Autodesk Fusion 360 part; units mm, degrees
sketch "Sketch1" plane through (0, 0, 0) normal (0, 0, 1) x (1, 0, 0)
  line L0 (0, 0) -> (129, 0)
  line L1 (129, 0) -> (129, 96.5)
  line L2 (129, 96.5) -> (0, 96.5)
  line L3 (0, 96.5) -> (0, 0)
  line L4 (3.25, 3.25) -> (125.75, 3.25)
  line L5 (125.75, 3.25) -> (125.75, 93.25)
  line L6 (125.75, 93.25) -> (3.25, 93.25)
  line L7 (3.25, 93.25) -> (3.25, 3.25)
  dimension "d1" = 129
  dimension "d2" = 96.5
  dimension "d3" = 122.5
  dimension "d4" = 90
  dimension "d5" = 3.25
  dimension "d6" = 3.25
extrude "Extrude1" add sketch "Sketch1" along normal blind 5
sketch "Sketch2" plane through (0, 0, 5) normal (0, 0, 1) x (-1, 0, 0)
  line L0 (-3.25, -3.25) -> (-3.25, -93.25)
  line L1 (-3.25, -93.25) -> (-125.75, -93.25)
  line L2 (-125.75, -93.25) -> (-125.75, -3.25)
  line L3 (-125.75, -3.25) -> (-3.25, -3.25)
  line L4 (0, -96.5) -> (0, 0)
  line L5 (0, 0) -> (-129, 0)
  line L6 (-129, 0) -> (-129, -96.5)
  line L7 (-129, -96.5) -> (0, -96.5)
  line L8 (-2, -2) -> (-127, -2)
  line L9 (-127, -2) -> (-127, -94.5)
  line L10 (-127, -94.5) -> (-2, -94.5)
  line L11 (-2, -94.5) -> (-2, -2)
  dimension "d9" = 125
  dimension "d10" = 92.5
  dimension "d11" = 2
  dimension "d12" = 2
extrude "Extrude2" cut sketch "Sketch2" against normal blind 2 contours L8 L9 L10 L11
move_face "OffsetFaces1" offset 50 1 faces at (84.9167, 1.0833, 0)
sketch "Sketch4" plane through (129, 0, 0) normal (1, 0, 0) x (0, 1, 0)
  line L0 (0, -50) -> (96.5, -50)
  line L1 (96.5, -50) -> (96.5, 5)
  line L2 (96.5, 5) -> (0, 5)
  line L3 (0, 5) -> (0, -50)
  line L4 (0, -50) -> (96.5, -50)
  line L5 (96.5, -50) -> (96.5, -52)
  line L6 (96.5, -52) -> (0, -52)
  line L7 (0, -52) -> (0, -50)
  dimension "d18" = 96.5
  dimension "d19" = 2
extrude "Extrude3" add sketch "Sketch4" against normal blind 129 contours L0 L4 L5 L6 L7
sketch "Sketch5" plane through (129, 0, 0) normal (1, 0, 0) x (0, 1, 0)
  line L0 (96.5, -52) -> (96.5, 5)
  line L1 (96.5, 5) -> (0, 5)
  line L2 (0, 5) -> (0, -52)
  line L3 (0, -52) -> (96.5, -52)
  line L4 (43.25, -52) -> (53.25, -52)
  line L5 (53.25, -52) -> (53.25, -50)
  line L6 (53.25, -50) -> (43.25, -50)
  line L7 (43.25, -50) -> (43.25, -52)
  dimension "d22" = 10
  dimension "d23" = 2
  dimension "d24" = 43.25
sketch "Sketch6" plane through (0, 0, 0) normal (-1, 0, 0) x (0, -1, 0)
  line L0 (0, -52) -> (0, 5)
  line L1 (0, 5) -> (-96.5, 5)
  line L2 (-96.5, 5) -> (-96.5, -52)
  line L3 (-96.5, -52) -> (0, -52)
  line L4 (-53.25, -52) -> (-43.25, -52)
  line L5 (-43.25, -52) -> (-43.25, -50)
  line L6 (-43.25, -50) -> (-53.25, -50)
  line L7 (-53.25, -50) -> (-53.25, -52)
  dimension "d25" = 10
  dimension "d26" = 2
  dimension "d27" = 43.25
extrude "Extrude4" add sketch "Sketch6" along normal blind 10 contours L3 L4 L5 L6 L7
extrude "Extrude5" add sketch "Sketch5" along normal blind 10 contours L3 L4 L5 L6 L7
sketch "Sketch7" plane through (0, 0, -50) normal (0, 0, 1) x (-1, 0, 0)
  line L0 (0, -43.25) -> (0, -53.25)
  line L1 (0, -53.25) -> (10, -53.25)
  line L2 (10, -53.25) -> (10, -43.25)
  line L3 (10, -43.25) -> (0, -43.25)
  circle A0 centre (5, -48.25) radius 3
  dimension "d32" = 6
  dimension "d33" = 5
  dimension "d34" = 5
extrude "Extrude6" cut sketch "Sketch7" against normal blind 2 contours A0
sketch "Sketch8" plane through (0, 0, -50) normal (0, 0, 1) x (-1, 0, 0)
  line L0 (-129, -53.25) -> (-129, -43.25)
  line L1 (-129, -43.25) -> (-139, -43.25)
  line L2 (-139, -43.25) -> (-139, -53.25)
  line L3 (-139, -53.25) -> (-129, -53.25)
  circle A0 centre (-134, -48.25) radius 3
  dimension "d37" = 6
  dimension "d38" = 5
  dimension "d39" = 5
extrude "Extrude7" cut sketch "Sketch8" against normal blind 2 contours A0
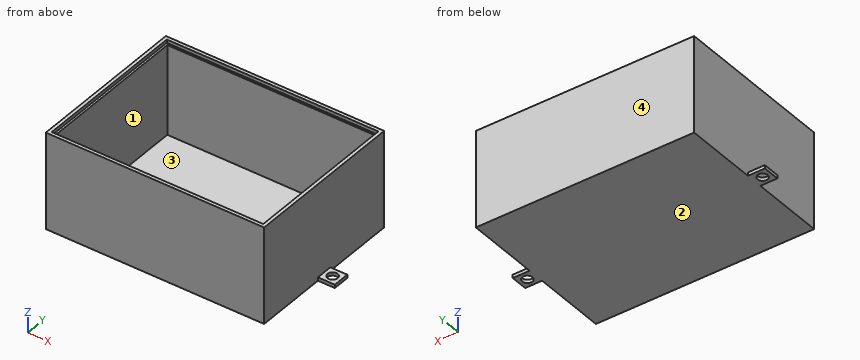
Input: part model. Units: mm. Frame: model coordinates. Face numbers are marked on the shaded views. A direction names the side the tool comes from. Coordinates: 2 decimals unless noted, no trailing zeros. Order: outer loops, then holes, each group sorted by start corner. A loop starts at its lowest first (then second) coordinate and runs counter-clockwise, first axis right, second up. Notation, with made-up numbers: M -9.5,13.5 L 31.5,13.5 A7 ccw 31.5,21.5 Z; hole C 12.25,26 d3. An arc over 180 degrees is marked long. Write item = value, one per line. Start each with the question number.
(1) Section C-C on z = -46. Output: boundary loops of the cut face in (x, y).
(2) Line query: line 1 along X through (y, z) = (48.25, -50.75); line 2 along X through (y, z) = (19, -9); line 3 along Y through (x, z) = (134, -50.85). Output: solid intervals per line, ascending. Write a range as [from, to].
(3) Reachability of the marked faces 3 and 4 from +Z, -Z, +X, -X, +Y, -Y: full face, straight path, thin tool, end or side. Return the list, or none.
(4) First-contact query: P1, Ø9.5, axis at x = 134, y = 48.25, coming from the +Z side; P2, Ø2, axis at y = 66, z = 3.5, coming from the +X side; P3, Ø2, axis at y = 64.5, z = -25, coming from the -X side. Flat tips, straight axial feed; report the tip coordinate or a pass-through.
(5) Section A-A on x = -5. Output: boundary loops of the cut face in (y, z).
(6) Pull-direction query (X, two-part tool) for the marked faces 1 and 2; classes: released by +X, released by -X, zero draft, split by the parting line, or undercut.
(7) Section B-B on y = 48.25. Output: boundary loops of the cut face in (x, z), and give its area (4 significant figures).
(8) Section D-D on x = 37.5. Output: boundary loops of the cut face in (y, z).
Result set:
q1.outline = M 0,0 L 129,0 L 129,96.5 L 0,96.5 Z; hole M 3.25,3.25 L 125.75,3.25 L 125.75,93.25 L 3.25,93.25 Z
q2.line_1 = [-10, -8], [-2, 131], [137, 139]
q2.line_2 = [0, 3.25], [125.75, 129]
q2.line_3 = [43.25, 45.25], [51.25, 53.25]
q3.face_3 = +Z
q3.face_4 = +Z, -Z, +X, -X, +Y
q4.P1 = -50
q4.P2 = 129
q4.P3 = 0
q5.outline = M 43.25,-52 L 45.25,-52 L 45.25,-50 L 43.25,-50 Z; M 51.25,-52 L 53.25,-52 L 53.25,-50 L 51.25,-50 Z
q6.face_1 = undercut
q6.face_2 = zero draft
q7.outline = M -10,-52 L -8,-52 L -8,-50 L -10,-50 Z; M -2,-52 L 131,-52 L 131,-50 L 129,-50 L 129,5 L 127,5 L 127,3 L 125.75,3 L 125.75,-50 L 3.25,-50 L 3.25,3 L 2,3 L 2,5 L 0,5 L 0,-50 L -2,-50 Z; M 137,-52 L 139,-52 L 139,-50 L 137,-50 Z
q7.area = 626.5 mm²
q8.outline = M 0,-52 L 96.5,-52 L 96.5,5 L 94.5,5 L 94.5,3 L 93.25,3 L 93.25,-50 L 3.25,-50 L 3.25,3 L 2,3 L 2,5 L 0,5 Z
